from build123d import *
from build123d import SkipClean  # not in build123d's __all__

# Parameters (mm, degrees)
F1_DEPTH      = 22
F2_R          = 8.15
F3_DEPTH      = 22.001
F3_TAPER      = 5.72
F4_W          = 40
F4_H          = 50
F5_DEPTH      = 12.5
F5_DEPTH_BACK = 34.5
F6_R          = 12.7
F7_DEPTH      = 40.001
F8_R          = 12.7
F9_DEPTH      = 10
F10_R         = 2.5
F11_DEPTH     = 25
F14_R         = 0.5
F15_DEPTH     = 2000


# Not quite as in the source:
# - after a boolean that leaves OpenCascade's solid faulty, fix() repairs it


with BuildPart() as f1:
    # F0 (on Front) → F1 (new body)
    with BuildSketch(Plane.XZ):
        with BuildLine():
            Line((0, 385), (0, 0))
            Line((0, 0), (40, 0))
            Line((40, 0), (40, 385))
            ThreePointArc((40, 385), (34.1421356237, 399.1421356237), (20, 405))
            ThreePointArc((20, 405), (5.8578643763, 399.1421356237), (0, 385))
        make_face()
    extrude(amount=F1_DEPTH)

    # F2 (on face) → F3 (cut, through all)
    with BuildSketch(Plane.XZ.offset(22)):
        with Locations((20, 385)):
            Circle(F2_R)
    extrude(amount=-F3_DEPTH, taper=F3_TAPER, mode=Mode.SUBTRACT)

    # F4 (on face) → F5 (join, two sides)
    with BuildSketch(Plane.XZ.offset(22)) as f5_sk:
        with Locations((20, 25)):
            Rectangle(F4_W, F4_H)
    extrude(amount=F5_DEPTH)
    extrude(f5_sk.sketch, amount=-F5_DEPTH_BACK)

    # F6 (on face) → F7 (cut, through all)
    with BuildSketch(Plane(origin=(0, 0, 0), x_dir=(0, -1, 0), z_dir=(-1, 0, 0))):
        with Locations((10, 25)):
            Circle(F6_R)
    extrude(amount=-F7_DEPTH, mode=Mode.SUBTRACT)

    # F8 (on face) → F9 (join)
    with BuildSketch(Plane.YZ.offset(40)):
        Polygon((0, 50), (-22, 50), (-34.5, 50), (-34.5, 0), (12.5, 0), (12.5, 50), align=None)
        with Locations((-10, 25)):
            Circle(F8_R, mode=Mode.SUBTRACT)
    with SkipClean():  # cleaning this boolean's faces spoils the solid; the shape is the same uncleaned
        extrude(amount=F9_DEPTH)

    # F10 (on face) → F11 (cut)
    with BuildSketch(Plane.XZ.offset(22)):
        with Locations((20, 55)):
            Circle(F10_R)
    extrude(amount=-F11_DEPTH, mode=Mode.SUBTRACT)

    add(f1.part.fix(), mode=Mode.REPLACE)

    # F14 (on line) → F15 (join)
    with BuildSketch(Plane(origin=(0, -26.8080383352, 393.2344937713), x_dir=(1, 0, 0), z_dir=(0, -0.0680152907, 0.9976842788))):
        with Locations((48.9524379373, -8.5178036243)):
            Circle(F14_R)
    extrude(amount=-F15_DEPTH)


solid = f1.part
Check sheet for the modelled part. Datum: model origin and axes. Units: mm. A direction names the side the tool comes from. Round coordinates to 2 decimals unless told otherwise and drop trailing zeros. Put each result on its own line as item: value. Start each with the question number.
1. Gauge pin test, flat ends, axial feed: pin 1 (4 mm diameter, centred on x = 33.5, z = 174, fed in from -Y); pin 2 (6.5 mm diameter, centred on y = -11.5, z = 177, fed in from +X); pin 3 (20.5 mm diameter, centred on y = -10, z = 25, fed in from -X). Record the tip position at first contact, or that the pin passes through.
2. Access from +Z, -Z, +X, -X, +Y, -Y to the whole of each face (thin tool, end or side, straight path). Record for faces 1 (the face through (20, 0, 230)), 2 (the face through (50, -22, 31)).
3. Scan lines: probe 1 along Y at (x, z) = (43.75, 25); probe 2 along Z at (x, y) = (20, -10); probe 3 along Y at (x, z) = (37, 214.5). Record each from-to range of solid material in increasing order.
Findings:
1. pin 1: stops at y = -22
1. pin 2: stops at x = 40
1. pin 3: stops at x = 48.45
2. face 1: +Z, +X, -X, +Y
2. face 2: +Z, -Z, +X, +Y, -Y
3. probe 1: y = -34.5 to -22.7, 2.7 to 12.5
3. probe 2: z = 0 to 12.3, 37.7 to 52.5, 57.5 to 378.05, 391.95 to 405
3. probe 3: y = -22 to 0
